```python
from build123d import *


with BuildPart() as part:
    # Sketch2 → Revolve1 (revolve)
    with BuildSketch(Plane(origin=(0, 0, 0), x_dir=(0, 0, -1), z_dir=(1, 0, 0))):
        with BuildLine():
            Line((12, 0), (12, 2.5))
            ThreePointArc((12, 2.5), (9.932956508, 3.306139112), (8.5, 5))
            Line((8.5, 5), (7, 5))
            Line((7, 5), (7, 2.5))
            Line((7, 2.5), (3, 2.5))
            Line((3, 2.5), (3, 0))
            Line((3, 0), (12, 0))
        make_face()
    revolve(axis=Axis((0, 0, 0), (0, 1, 0)))


solid = part.part
```
The listing builds one solid part. Answer for the finished solid, in the listing's coordinates (mm). A direction names the side the tool comes from. Round coordinates to 2 decimals unless told otherwise and drop trailing zeros. Order: outer loops, then holes, each group sorted by start corner. A loop starts at its lowest first (then second) coordinate and runs counter-clockwise, first axis right, second up. Notation, with made-up numbers: (-3, -25) -> (7, -25) arc R31 cw to (7, 5) -> close; hole circle Ø4 at (1, 43). An arc over 180 degrees is marked (long way). Answer as CSV lines item,"result". Start each with the question number.
(1) For a pull along Z with two mould halves and no side action, classify faces 3 (the face through (0, 1, 3)), 4 (the face through (2.5, 0, 2.5)), 5 (the face through (-0.53, 1.27, 11.99)) as +Z half, -Z half, draft (parallel to the pull), parting line (faces both ways), or undercut.
(2) The part is cut by section A-A (x = 0). Determine the outline of the cut face in (y, z), then the cut area to 3 significant figures.
(3) Find the intervals of material crossed by probe 1 along Z at (x, y) = (0, 1); probe 2 along X at (y, z) = (3.5, 0), in increasing order. Write a range as from..to.
(4) Flat-ended cylindrical pins translate along their axes: pin 1 Ø1.5 at (x, y) = (6.5, 4) entering from -Z; pin 2 Ø2 at (x, y) = (-4.5, 0.5) entering from +Z; pin 3 Ø11 at (x, z) = (-0.5, 1) entering from +Y. Find the tip coordinate at first contact, or state that the pin passes through.
(5) The part is cut by section D-D (y = 3.3). Determine the outline of the cut face in (x, z).
(6) The part is cut by section C-C (y = 0.5). Determine the outline of the cut face in (x, z), then the cut area to 3 significant figures.
(7) A tool of negligible diameter and unlimited length cuts with its end or side. For faces 1 (the face through (3, 2.5, -1)), 2 (the face through (-7, 5, -2)), from which of +Z, -Z, +X, -X, +Y, -Y can it reach the whole face along a straight path? Write none if from no direction.
(8) The part is cut by section B-B (z = 0). Determine the outline of the cut face in (x, y), then the cut area to 3 significant figures.
Evaluation:
1,face 3,"undercut"
1,face 4,"draft"
1,face 5,"parting line"
2,outline,"(0, -12) -> (2.5, -12) arc R4.51 cw to (5, -8.5) -> (5, -7) -> (2.5, -7) -> (2.5, -3) -> (0, -3) -> close; (0, 3) -> (2.5, 3) -> (2.5, 7) -> (5, 7) -> (5, 8.5) arc R4.51 cw to (2.5, 12) -> (0, 12) -> close"
2,area,"58.1 mm²"
3,probe 1,"-12..-3, 3..12"
3,probe 2,"-9.68..-7, 7..9.68"
4,pin 1,"z = -7.75"
4,pin 2,"z = 11.48"
4,pin 3,"y = 2.5"
5,outline,"circle Ø19.88 at (0, 0); hole circle Ø14 at (0, 0)"
6,outline,"circle Ø24 at (0, 0); hole circle Ø6 at (0, 0)"
6,area,"424 mm²"
7,face 1,"+Y"
7,face 2,"+Z, -Z, +X, -X, +Y"
8,outline,"(-12, 0) -> (-3, 0) -> (-3, 2.5) -> (-7, 2.5) -> (-7, 5) -> (-8.5, 5) arc R4.51 cw to (-12, 2.5) -> close; (3, 0) -> (12, 0) -> (12, 2.5) arc R4.51 cw to (8.5, 5) -> (7, 5) -> (7, 2.5) -> (3, 2.5) -> close"
8,area,"58.1 mm²"
